from build123d import *

# Parameters (mm, degrees)
BOSS_EXTRUDE1_DEPTH = 3.175
SKETCH3_R           = 1.27
CUT_EXTRUDE1_DEPTH  = 90.413321575
CUT_EXTRUDE2_START  = -3.175
CUT_EXTRUDE2_DEPTH  = 3.175


# Read off the part's stored shape, not the designer's step: Cut-Extrude2
with BuildPart() as part:
    # Sketch2 → Boss-Extrude1 (new body)
    with BuildSketch(Plane(origin=(0, 0, 0), x_dir=(1, 0, 0), z_dir=(0, 1, 0))):
        with BuildLine():
            Line((6.35, 56.515), (56.515, 56.515))
            Line((56.515, 56.515), (56.515, -56.515))
            Line((56.515, -56.515), (12.7, -56.515))
            ThreePointArc((12.7, -56.515), (0, -69.215), (-12.7, -56.515))
            Line((-12.7, -56.515), (-56.515, -56.515))
            Line((-56.515, -56.515), (-56.515, 56.515))
            Line((-56.515, 56.515), (-6.35, 56.515))
            Line((-6.35, 56.515), (-6.35, -50.165))
            Line((-6.35, -50.165), (6.35, -50.165))
            Line((6.35, -50.165), (6.35, 56.515))
        make_face()
    extrude(amount=BOSS_EXTRUDE1_DEPTH)

    # Sketch3 → Cut-Extrude1 (cut, through all)
    with BuildSketch(Plane(origin=(0, 3.175, 0), x_dir=(1, 0, 0), z_dir=(0, 1, 0))):
        with Locations(Location((0, -62.865, 0), (0, 0, 270))):
            Circle(SKETCH3_R)
    extrude(amount=-CUT_EXTRUDE1_DEPTH, mode=Mode.SUBTRACT)

    # Cut-Extrude2 outline → Cut-Extrude2 (cut)
    with BuildSketch(Plane(origin=(0, 3.175, 0), x_dir=(1, 0, 0), z_dir=(0, 1, 0)).offset(CUT_EXTRUDE2_START)):
        with BuildLine():
            ThreePointArc((6.35, 56.157125327), (42.147452325, 37.650199037), (56.515, 0))
            Line((56.515, 0), (56.515, 56.515))
            Line((56.515, 56.515), (6.35, 56.515))
            Line((6.35, 56.515), (6.35, 56.157125327))
        make_face()
        with BuildLine():
            ThreePointArc((56.515, 0), (44.224912238, -35.186678765), (12.7, -55.069548981))
            Line((12.7, -55.069548981), (12.7, -56.515))
            Line((12.7, -56.515), (56.515, -56.515))
            Line((56.515, -56.515), (56.515, 0))
        make_face()
        with BuildLine():
            ThreePointArc((-12.7, -55.069548981), (-44.224912408, -35.186678552), (-56.515, 5.45e-07))
            Line((-56.515, 5.45e-07), (-56.515, -56.515))
            Line((-56.515, -56.515), (-12.7, -56.515))
            Line((-12.7, -56.515), (-12.7, -55.069548981))
        make_face()
        with BuildLine():
            ThreePointArc((-56.515, 5.45e-07), (-42.147452144, 37.65019924), (-6.35, 56.157125327))
            Line((-6.35, 56.157125327), (-6.35, 56.515))
            Line((-6.35, 56.515), (-56.515, 56.515))
            Line((-56.515, 56.515), (-56.515, 5.45e-07))
        make_face()
    extrude(amount=CUT_EXTRUDE2_DEPTH, mode=Mode.SUBTRACT)


solid = part.part
Model file for the job. Use its own axes, mm. A direction names the side the tool comes from. Give positions to 0.01 mm unless a question says otherwise; leave off trailing zeros. Loops run counter-clockwise (first coordinate to the right, second up) from the corner with the lowest first, then second, coordinate; pieces in that order, holes last. Notation, with made-up numbers: (64.25, 57.25) - (100.25, 57.25) arc R27 cw to (100.25, 93.25) - close; hole circle Ø4 at (63, 11). An arc over 180 degrees is marked (long way). Use one line per item in the form item = value.
(1) Pull direction Z, two halves, no side cores. Call faces 1 (the face through (0.28, 1.57, 69.21)), 2 (the face through (-0.486, 1.61, 64.038)), 3 (the face through (-12, 3.175, 6)): pulls with the +Z half, pulls with the -Z half, needs draft (parallel to the pull), parting line crosses it, or undercut.
Determined:
face_1 = pulls with the +Z half
face_2 = undercut
face_3 = needs draft
(2) Cut at A-A (z = -7). Give the cut face in (x, y) (3 decimals), then the cut area to 3 significant figures.
Determined:
outline = (-56.08, 0) - (-6.35, 0) - (-6.35, 3.175) - (-56.08, 3.175) - close; (6.35, 0) - (56.08, 0) - (56.08, 3.175) - (6.35, 3.175) - close
area = 316 mm^2
(3) 3-axis set-ups, long thin cutter, end or side, ignore diameter. For faces 4 (the face through (6.35, 2, -2)), 5 (the face through (-12, 0, 6)): which of +Z, -Z, +X, -X, +Y, -Y reach the whole face in a straight line?
Determined:
face_4 = -Z, +Y, -Y
face_5 = +Z, -Z, +X, -X, -Y
(4) Cut at B-B (y = 1.7). Give the cut face in (x, z) (3 decimals).
Determined:
outline = (-12.7, 55.07) arc R56.515 ccw to (-6.35, -56.157) - (-6.35, 50.165) - (6.35, 50.165) - (6.35, -56.157) arc R56.515 ccw to (12.7, 55.07) - (12.7, 56.515) arc R12.7 ccw to (-12.7, 56.515) - close; hole circle Ø2.54 at (0, 62.865)
(5) Cut at C-C (z = 15.5). Give the cut face in (x, y) (3 decimals), then the cut area to 3 significant figures.
Determined:
outline = (-54.348, 0) - (-6.35, 0) - (-6.35, 3.175) - (-54.348, 3.175) - close; (6.35, 0) - (54.348, 0) - (54.348, 3.175) - (6.35, 3.175) - close
area = 305 mm^2
(6) Drop flat-ended pins along their axis: P1, Ø1.5, axis at x = 0, z = 62.865, coming from the -Y side; P2, Ø1.6, axis at x = 1, y = 1.5, coming from the -Z side (3 decimals); P3, Ø1.6, axis at y = 1.5, z = 5, coming from the -X side; P4, Ø1, axis at y = 1, z = -11.5, coming from the -X side. Give the stop position or say it passes through.
Determined:
P1 = through
P2 = 50.165
P3 = -56.36
P4 = -55.43
(7) Drill centre lines: L1, parallel to X at y = 1.2, z = 0 (3 decimals); L2, parallel to X at y = 2.55, z = -26.5; L3, parallel to X at y = 2.25, z = 60. Where is each one in solid material? Low to high.
Determined:
L1 = -56.515 to -6.35, 6.35 to 56.515
L2 = -49.92 to -6.35, 6.35 to 49.92
L3 = -12.21 to 12.21
(8) Cut at D-D (x = 29). Give the cut face in (y, z) (3 decimals), then the cut area to 3 significant figures.
Determined:
outline = (0, -48.507) - (3.175, -48.507) - (3.175, 48.507) - (0, 48.507) - close
area = 308 mm^2
